The model under review builds one solid part; all positions refer to its coordinate system, in mm. Coordinates: 2 decimals unless noted, no trailing zeros. Write each loop counter-clockwise with the first axis right and the second up, starting at its lowest first coordinate (ties: lowest second). Pieces come first, ordered by that corner, then holes. Notation, with made-up numbers: (-3.5, -22) - (39.5, -22) arc R27 ccw to (39.5, 3) - close; hole circle Ø8 at (47.5, 33.25). An arc over 180 degrees is marked (long way). Put each result on its own line as item: value.
from build123d import *

# Parameters (mm, degrees)
SKETCH1_W               = 140
SKETCH1_H               = 87
BOSS_EXTRUDE1_DEPTH     = 4
BOSS_EXTRUDE2_START     = -4
BOSS_EXTRUDE2_OUTLINE_R = 2
BOSS_EXTRUDE2_DEPTH     = 4
FILLET1_R               = 5


# Read off the part's stored shape, not the designer's step: Boss-Extrude2
with BuildPart() as part:
    # Sketch1 → Boss-Extrude1 (new body)
    with BuildSketch(Plane(origin=(0, 0, 0), x_dir=(1, 0, 0), z_dir=(0, 1, 0))):
        Rectangle(SKETCH1_W, SKETCH1_H)
    extrude(amount=BOSS_EXTRUDE1_DEPTH)

    # Boss-Extrude2 outline → Boss-Extrude2 (cut)
    with BuildSketch(Plane(origin=(0, 4, 0), x_dir=(1, 0, 0), z_dir=(0, 1, 0)).offset(BOSS_EXTRUDE2_START)):
        with Locations((-65.5, 35)):
            Circle(BOSS_EXTRUDE2_OUTLINE_R)
        with Locations((65.5, -35)):
            Circle(BOSS_EXTRUDE2_OUTLINE_R)
        with Locations((-65.5, -35)):
            Circle(BOSS_EXTRUDE2_OUTLINE_R)
        with Locations((65.5, 35)):
            Circle(BOSS_EXTRUDE2_OUTLINE_R)
    extrude(amount=BOSS_EXTRUDE2_DEPTH, mode=Mode.SUBTRACT)

    # Fillet1
    fillet1_edges = [part.edges().sort_by_distance(p)[0] for p in [
        (70, 2, 43.5),
        (-70, 2, 43.5),
        (-70, 2, -43.5),
        (70, 2, -43.5),
    ]]
    fillet(fillet1_edges, radius=FILLET1_R)


solid = part.part
1. To check wall thickness, follow probe 1 along Z at (x, y) = (65.5, 2.9); probe 2 along X at (y, z) = (1.3, -35). State the ranges of each line that lie inside material, in increasing order.
Determined:
probe 1: z = -43.47 to -37, -33 to 33, 37 to 43.47
probe 2: x = -70 to -67.5, -63.5 to 63.5, 67.5 to 70
2. The part is to be moulded in two halves that separate along X. For faces 1 (the flat face through (-1, 2, -43.5)), 2 (the cylindrical face through (-65.934, 1.972, 36.952)), 3 (the cylindrical face through (68.5, 2.03, 42.07)), 4 (the cylindrical face through (65.066, 1.972, 36.952)), say which applies: +X half, -X half, draft (parallel to the pull), parting line (faces both ways), or undercut.
Determined:
face 1: draft
face 2: undercut
face 3: +X half
face 4: undercut
3. For pin 1 Ø2.5 at (x, z) = (65.5, -35) entering from +Y, flat-tipped, find the tip position at first contact; note if it passes through.
Determined:
pin 1: passes through
4. Consider section A-A on z = -35. State the section outline as (x, y) points, plus the area to 3 significant figures.
Determined:
outline: (-70, 0) - (-67.5, 0) - (-67.5, 4) - (-70, 4) - close; (-63.5, 0) - (63.5, 0) - (63.5, 4) - (-63.5, 4) - close; (67.5, 0) - (70, 0) - (70, 4) - (67.5, 4) - close
area: 528 mm^2
